```python
from build123d import *

# Parameters (mm, degrees)
SKETCH_1_R           = 0.9
EXTRUDE_1_DEPTH      = 1.5
SKETCH_2_W           = 13.8
SKETCH_2_H           = 24.6
EXTRUDE_2_DEPTH      = 1.5
SKETCH_3_W           = 3.7
SKETCH_3_H           = 6
EXTRUDE_3_DEPTH      = 1.4
SKETCH_4_W           = 1.3
SKETCH_4_H           = 2.5
EXTRUDE_4_DEPTH      = 1.2
CHAMFER_1_SIZE       = 0.5
EXTRUDE_5_DEPTH      = 1.2
EXTRUDE_5_DEPTH_BACK = 9.5
SKETCH_5_R           = 0.4
SKETCH_6_W           = 2.4
SKETCH_6_H           = 20.18
SKETCH_6_R           = 0.4
EXTRUDE_6_DEPTH      = 2


with BuildPart() as part:
    # Эскиз1 → Бобышка-Вытянуть1 (new body)
    with BuildSketch(Plane(origin=(0, 0, 0), x_dir=(1, 0, 0), z_dir=(0, 1, 0))):
        with BuildLine():
            Line((11.75, 22.2), (-11.75, 22.2))
            ThreePointArc((-11.75, 22.2), (-13.164213562, 21.614213562), (-13.75, 20.2))
            Line((-13.75, 20.2), (-13.75, -20.2))
            ThreePointArc((-13.75, -20.2), (-13.164213562, -21.614213562), (-11.75, -22.2))
            Line((-11.75, -22.2), (11.75, -22.2))
            ThreePointArc((11.75, -22.2), (13.164213562, -21.614213562), (13.75, -20.2))
            Line((13.75, -20.2), (13.75, 20.2))
            ThreePointArc((13.75, 20.2), (13.164213562, 21.614213562), (11.75, 22.2))
        make_face()
        with Locations(Location((11.35, 19.8, 0), (0, 0, 270))):
            Circle(SKETCH_1_R, mode=Mode.SUBTRACT)
        with Locations(Location((-11.35, 19.8, 0), (0, 0, 270))):
            Circle(SKETCH_1_R, mode=Mode.SUBTRACT)
        with Locations(Location((-11.35, -19.8, 0), (0, 0, 90))):
            Circle(SKETCH_1_R, mode=Mode.SUBTRACT)
        with Locations(Location((11.35, -19.8, 0), (0, 0, 90))):
            Circle(SKETCH_1_R, mode=Mode.SUBTRACT)
    extrude(amount=EXTRUDE_1_DEPTH)

    # Эскиз2 → Бобышка-Вытянуть2 (add)
    with BuildSketch(Plane(origin=(0, 1.5, 0), x_dir=(1, 0, 0), z_dir=(0, 1, 0))):
        with Locations((-0.25, 4.2)):
            Rectangle(SKETCH_2_W, SKETCH_2_H)
    extrude(amount=EXTRUDE_2_DEPTH)

    # Эскиз3 → Бобышка-Вытянуть3 (add)
    with BuildSketch(Plane(origin=(0, 1.5, 0), x_dir=(1, 0, 0), z_dir=(0, 1, 0))):
        with Locations((8.5, -14.2)):
            Rectangle(SKETCH_3_W, SKETCH_3_H)
        with Locations((2.8, -14.2)):
            Rectangle(SKETCH_3_W, SKETCH_3_H)
        with Locations((-2.8, -14.2)):
            Rectangle(SKETCH_3_W, SKETCH_3_H)
        with Locations((-8.3, -14.2)):
            Rectangle(SKETCH_3_W, SKETCH_3_H)
    extrude(amount=EXTRUDE_3_DEPTH)

    # Эскиз4 → Бобышка-Вытянуть4 (add)
    with BuildSketch(Plane(origin=(0, 2.9, 0), x_dir=(1, 0, 0), z_dir=(0, 1, 0))):
        with Locations((8.5, -14.2)):
            Rectangle(SKETCH_4_W, SKETCH_4_H)
        with Locations((2.8, -14.2)):
            Rectangle(SKETCH_4_W, SKETCH_4_H)
        with Locations((-2.8, -14.2)):
            Rectangle(SKETCH_4_W, SKETCH_4_H)
        with Locations((-8.3, -14.2)):
            Rectangle(SKETCH_4_W, SKETCH_4_H)
    extrude(amount=EXTRUDE_4_DEPTH)

    # Фаска1
    chamfer_1_edges = [part.edges().sort_by_distance(p)[0] for p in [
        (9.15, 2.9, 14.2),
        (8.5, 2.9, 12.95),
        (7.85, 2.9, 14.2),
        (8.5, 2.9, 15.45),
        (2.8, 2.9, 12.95),
        (2.15, 2.9, 14.2),
        (2.8, 2.9, 15.45),
        (3.45, 2.9, 14.2),
        (-2.8, 2.9, 12.95),
        (-3.45, 2.9, 14.2),
        (-2.8, 2.9, 15.45),
        (-2.15, 2.9, 14.2),
        (-8.3, 2.9, 12.95),
        (-8.95, 2.9, 14.2),
        (-8.3, 2.9, 15.45),
        (-7.65, 2.9, 14.2),
    ]]
    chamfer(chamfer_1_edges, length=CHAMFER_1_SIZE)

    # Эскиз5 → Бобышка-Вытянуть5 (add, two sides: drawn at the far end of the back side and taken through both)
    with BuildSketch(Plane(origin=(0, 1.5, 0), x_dir=(1, 0, 0), z_dir=(0, 1, 0)).offset(-EXTRUDE_5_DEPTH_BACK)):
        with Locations(Location((12.15, 9.5, 0), (0, 0, 270))):
            Circle(SKETCH_5_R)
        with Locations(Location((12.15, 6.96, 0), (0, 0, 270))):
            Circle(SKETCH_5_R)
        with Locations(Location((12.15, 4.42, 0), (0, 0, 270))):
            Circle(SKETCH_5_R)
        with Locations(Location((12.15, 1.88, 0), (0, 0, 270))):
            Circle(SKETCH_5_R)
        with Locations(Location((12.15, -0.66, 0), (0, 0, 270))):
            Circle(SKETCH_5_R)
        with Locations(Location((12.15, -3.2, 0), (0, 0, 270))):
            Circle(SKETCH_5_R)
        with Locations(Location((12.15, -5.74, 0), (0, 0, 270))):
            Circle(SKETCH_5_R)
        with Locations(Location((12.15, -8.28, 0), (0, 0, 270))):
            Circle(SKETCH_5_R)
    extrude(amount=EXTRUDE_5_DEPTH + EXTRUDE_5_DEPTH_BACK)

    # Эскиз6 → Бобышка-Вытянуть6 (add)
    with BuildSketch(Plane.XZ):
        with Locations((12.15, -0.61)):
            Rectangle(SKETCH_6_W, SKETCH_6_H)
        with Locations(Location((12.15, -9.5, 0), (0, 0, 90))):
            Circle(SKETCH_6_R, mode=Mode.SUBTRACT)
        with Locations(Location((12.15, -6.96, 0), (0, 0, 90))):
            Circle(SKETCH_6_R, mode=Mode.SUBTRACT)
        with Locations(Location((12.15, -4.42, 0), (0, 0, 90))):
            Circle(SKETCH_6_R, mode=Mode.SUBTRACT)
        with Locations(Location((12.15, -1.88, 0), (0, 0, 90))):
            Circle(SKETCH_6_R, mode=Mode.SUBTRACT)
        with Locations(Location((12.15, 0.66, 0), (0, 0, 90))):
            Circle(SKETCH_6_R, mode=Mode.SUBTRACT)
        with Locations(Location((12.15, 3.2, 0), (0, 0, 90))):
            Circle(SKETCH_6_R, mode=Mode.SUBTRACT)
        with Locations(Location((12.15, 5.74, 0), (0, 0, 90))):
            Circle(SKETCH_6_R, mode=Mode.SUBTRACT)
        with Locations(Location((12.15, 8.28, 0), (0, 0, 90))):
            Circle(SKETCH_6_R, mode=Mode.SUBTRACT)
    extrude(amount=EXTRUDE_6_DEPTH)


solid = part.part
```
Can you work these out from the model? Positions are in its coordinate system, mm. A direction names the side the tool comes from. Coordinates: 2 decimals unless noted, no trailing zeros. Order: outer loops, then holes, each group sorted by start corner. A loop starts at its lowest first (then second) coordinate and runs counter-clockwise, first axis right, second up. Notation, with made-up numbers: (60.25, 88.5) - (95.25, 88.5) arc R12 cw to (95.25, 93.5) - close; hole circle Ø3 at (-15, -18.5). An arc over 180 degrees is marked (long way). Answer in a Markdown table with one row per item.
1. If I drill on line 1 along X through (y, z) = (0.35, 19.8); line 2 along Z through (x, y) = (1.25, 1.75); line 3 along Y through (x, z) = (9.75, 0.5), over which ranges is the centre line in solid material (lowest first)?
Reply:
| item | result |
|---|---|
| line 1 | x = -13.75 to -12.25, -10.45 to 10.45, 12.25 to 13.75 |
| line 2 | z = -16.5 to 8.1, 11.2 to 17.2 |
| line 3 | y = 0 to 1.5 |
2. If we mould it in two halves opening along X, with no side actions, what happens to faces 1 (the flat face through (-4.65, 2, 14)), 2 (the flat face through (-7.15, 2, -4)), 3 (the flat face through (12, -2, 0))? For each: pulls with the +X half, pulls with the -X half, needs draft (parallel to the pull), parting line crosses it, or undercut.
Reply:
| item | result |
|---|---|
| face 1 | undercut |
| face 2 | pulls with the -X half |
| face 3 | needs draft |
3. For pin 1 (5 mm diameter, centred on x = -10.5, z = 16.5, fed in from -Y); pin 2 (0.6 mm diameter, centred on x = 2.5, y = 4, fed in from +Z); pin 3 (0.6 mm diameter, centred on y = 4, z = 14.5, fed in from -X), each with a flat end and sliding along its axis, tell me the tip position at first contact or that it passes through.
Reply:
| item | result |
|---|---|
| pin 1 | stops at y = 0 |
| pin 2 | stops at z = 15.45 |
| pin 3 | stops at x = -8.95 |
4. For faces 4 (the flat face through (-0.95, 2, 14)), 5 (the flat face through (10.95, -1, -1)), 6 (the flat face through (13.35, -1, -1)), which set-ups out of +Z, -Z, +X, -X, +Y, -Y let a thin tool reach every point of the face, with its end or its side?
Reply:
| item | result |
|---|---|
| face 4 | +Z, +Y |
| face 5 | +Z, -Z, -X, -Y |
| face 6 | +Z, -Z, +X, -Y |
5. Suppose I cut it at C-C (z = -3.5). Please give me the cut outline in (x, y), and give its area (4 significant figures).
Reply:
| item | result |
|---|---|
| outline | (-13.75, 0) - (10.95, 0) - (10.95, -2) - (13.35, -2) - (13.35, 0) - (13.75, 0) - (13.75, 1.5) - (6.65, 1.5) - (6.65, 3) - (-7.15, 3) - (-7.15, 1.5) - (-13.75, 1.5) - close |
| area | 66.75 mm^2 |
6. Suppose I cut it at A-A (y = -6.25). Please give me the cut outline in (x, z), and give its area (3 significant figures).
Reply:
| item | result |
|---|---|
| outline | circle Ø0.8 at (12.15, -9.5); circle Ø0.8 at (12.15, -6.96); circle Ø0.8 at (12.15, -4.42); circle Ø0.8 at (12.15, -1.88); circle Ø0.8 at (12.15, 0.66); circle Ø0.8 at (12.15, 3.2); circle Ø0.8 at (12.15, 5.74); circle Ø0.8 at (12.15, 8.28) |
| area | 4.02 mm^2 |
7. Suppose I cut it at B-B (x = -0.5). Please give me the cut outline in (y, z), and give its area (4 significant figures).
Reply:
| item | result |
|---|---|
| outline | (0, -22.2) - (1.5, -22.2) - (1.5, -16.5) - (3, -16.5) - (3, 8.1) - (1.5, 8.1) - (1.5, 22.2) - (0, 22.2) - close |
| area | 103.5 mm^2 |
